Source: CAD feature listing. Evaluate the final solid. Frame: model axes, mm. A direction names the side the tool comes from. Round coordinates to 2 decimals unless told otherwise and drop trailing zeros. Order: outer loops, then holes, each group sorted by start corner. A loop starts at its lowest first (then second) coordinate and runs counter-clockwise, first axis right, second up. Notation, with made-up numbers: (-6.5, -3) - (15.5, -3) arc R12 ccw to (15.5, 2) - close; hole circle Ø8 at (60, -32). An arc over 180 degrees is marked (long way). Use one line per item in the form item = value. Start each with the question number.
Q1. Cut plane A-A, the plane x = 48.2. Return the cut outline in (y, z), and give its area (3 significant figures).
Q2. Ray query, line 1 (Z direction, x = -5.3, y = 27.5); line 2 (X direction, y = 44.25, z = -9.6) (3 decimals); line 3 (Y direction, x = 5.5, z = -8). Return the intervals inside material, ascending. Write a range as [from, to].
Q3. Cut plane B-B, the plane x = 28. Return the cut outline in (y, z), and give its area (3 significant figures).
Q4. Draft query along X for faces 1 (the cylindrical face through (45.8, 26.82, -4.71)), 2 (the cylindrical face through (-2.9, 26.82, -14.31)), 3 (the flat face through (-8, 27, -3)), 4 (the flat face through (22, 38.7, -10)). Return one class per face: released by +X, released by -X, zero draft, split by the parting line, or undercut.
Q5. Cut plane D-D, the plane y = 23. Return the cut outline in (x, z), and give its area (3 significant figures).
Q6. Pin query (flat end, axial travel): pin 1 Ø1.7 at (x, z) = (10.725, -9.6) entering from +Y; pin 2 Ø2.5 at (y, z) = (37, -13) entering from +X; pin 3 Ø2 at (y, z) = (22.5, -4.5) entering from -X. Return the tip coordinate at first contact, or that it passes through.
Q7. Set-up query: faces 5 (the flat face through (16, 40.2, -13)), 6 (the flat face through (35.175, 37.5, -3.7)), 7 (the flat face through (47, 28.3, -10)). Return all of +Z, -Z, +X, -X, +Y, -Y with unobstructed straight access to the full face (end or side cutting, diameter ignored); none if empty.
from build123d import *

# Parameters (mm, degrees)
SKETCH_1_W             = 42.9
SKETCH_1_H             = 19.2
EXTRUDE_1_DEPTH        = 35.7
EXTRUDE_3_DEPTH        = 3
SKETCH_5_R             = 7.2
EXTRUDE_4_DEPTH        = 1.5
SKETCH_6_R             = 5.76
EXTRUDE_5_DEPTH        = 0.3
CUT_EXTRUDE_START      = -0.3
CUT_EXTRUDE_3_DEPTH    = 0.3
EXTRUDE_6_DEPTH        = 8
FILLET_1_R             = 2
FILLET_2_R             = 2
CUT_EXTRUDE_4_DEPTH    = 62.321611199
FILLET_1_OF_MIRROR_2_R = 2
FILLET_2_OF_MIRROR_2_R = 2
SKETCH_10_R            = 2.88
EXTRUDE_7_DEPTH        = 6
SKETCH_11_R            = 1.44
CUT_EXTRUDE_5_DEPTH    = 6


with BuildPart() as part:
    # Sketch 1 → Extrude 1 (new body)
    with BuildSketch(Plane(origin=(0, 0, 0), x_dir=(1, 0, 0), z_dir=(0, 1, 0))):
        with Locations((21.45, 9.6)):
            Rectangle(SKETCH_1_W, SKETCH_1_H)
    extrude(amount=EXTRUDE_1_DEPTH)

    # Sketch 2 → Extrude 3 (add)
    with BuildSketch(Plane(origin=(0, 35.7, 0), x_dir=(1, 0, 0), z_dir=(0, 1, 0))):
        with BuildLine():
            Line((35.175, 1), (35.175, 3.875))
            ThreePointArc((35.175, 3.875), (40.9, 9.6), (35.175, 15.325))
            Line((35.175, 15.325), (35.175, 18.2))
            Line((35.175, 18.2), (14.991145802, 18.2))
            ThreePointArc((14.991145802, 18.2), (1.125, 9.6), (14.991145802, 1))
            Line((14.991145802, 1), (35.175, 1))
        make_face()
    extrude(amount=EXTRUDE_3_DEPTH)

    # Sketch 5 → Extrude 4 (add)
    with BuildSketch(Plane(origin=(0, 38.7, 0), x_dir=(1, 0, 0), z_dir=(0, 1, 0))):
        with Locations(Location((10.725, 9.6, 0), (0, 0, 270))):
            Circle(SKETCH_5_R)
    extrude(amount=EXTRUDE_4_DEPTH)

    # Sketch 6 → Extrude 5 (add)
    with BuildSketch(Plane(origin=(0, 40.2, 0), x_dir=(1, 0, 0), z_dir=(0, 1, 0))):
        with Locations(Location((10.725, 9.6, 0), (0, 0, 270))):
            Circle(SKETCH_6_R)
    extrude(amount=EXTRUDE_5_DEPTH)

    # Sketch 4 → Cut-Extrude 3 (cut)
    with BuildSketch(Plane(origin=(0, 38.7, 0), x_dir=(1, 0, 0), z_dir=(0, 1, 0)).offset(CUT_EXTRUDE_START)):
        with BuildLine():
            Line((35.175, 15.325), (35.175, 3.875))
            ThreePointArc((35.175, 3.875), (40.9, 9.6), (35.175, 15.325))
        make_face()
    extrude(amount=CUT_EXTRUDE_3_DEPTH, mode=Mode.SUBTRACT)

    # Sketch 8 → Extrude 6 (add)
    with BuildSketch(Plane(origin=(42.9, 0, 0), x_dir=(0, 0, -1), z_dir=(1, 0, 0))):
        Polygon((19.2, 26.8), (19.2, 28.3), (0, 28.3), (0, 25.3), (19.2, 25.3), align=None)
    extrude_6 = extrude(amount=EXTRUDE_6_DEPTH)

    # Fillet 1
    fillet_1_edges = [part.edges().sort_by_distance(p)[0] for p in [
        (50.9, 26.8, 0),
    ]]
    fillet(fillet_1_edges, radius=FILLET_1_R)

    # Fillet 2
    fillet_2_edges = [part.edges().sort_by_distance(p)[0] for p in [
        (50.9, 26.8, -19.2),
    ]]
    fillet(fillet_2_edges, radius=FILLET_2_R)

    # Sketch 9 → Cut-Extrude 4 (cut, through all)
    with BuildSketch(Plane(origin=(0, 28.3, 0), x_dir=(1, 0, 0), z_dir=(0, 1, 0))):
        with BuildLine():
            Line((50.381742423, 5.8), (50.9, 5.8))
            Line((50.9, 5.8), (50.9, 3.8))
            Line((50.9, 3.8), (50.381742423, 3.8))
            ThreePointArc((50.381742423, 3.8), (45.8, 4.8), (50.381742423, 5.8))
        make_face()
        with BuildLine():
            Line((50.381742423, 15.4), (50.9, 15.4))
            Line((50.9, 15.4), (50.9, 13.4))
            Line((50.9, 13.4), (50.381742423, 13.4))
            ThreePointArc((50.381742423, 13.4), (45.8, 14.4), (50.381742423, 15.4))
        make_face()
    cut_extrude_4 = extrude(amount=-CUT_EXTRUDE_4_DEPTH, mode=Mode.SUBTRACT)

    # Mirror 2: Extrude 6, Cut-Extrude 4 across plane
    add(extrude_6.mirror(Plane(origin=(21.45, 0, 0), x_dir=(0, 0, 1), z_dir=(1, 0, 0))))
    add(cut_extrude_4.mirror(Plane(origin=(21.45, 0, 0), x_dir=(0, 0, 1), z_dir=(1, 0, 0))), mode=Mode.SUBTRACT)

    # Fillet 1 of Mirror 2
    fillet_1_of_mirror_2_edges = [part.edges().sort_by_distance(p)[0] for p in [
        (-8, 26.8, 0),
    ]]
    fillet(fillet_1_of_mirror_2_edges, radius=FILLET_1_OF_MIRROR_2_R)

    # Fillet 2 of Mirror 2
    fillet_2_of_mirror_2_edges = [part.edges().sort_by_distance(p)[0] for p in [
        (-8, 26.8, -19.2),
    ]]
    fillet(fillet_2_of_mirror_2_edges, radius=FILLET_2_OF_MIRROR_2_R)

    # Sketch 10 → Extrude 7 (add)
    with BuildSketch(Plane(origin=(0, 40.5, 0), x_dir=(1, 0, 0), z_dir=(0, 1, 0))):
        with Locations(Location((10.725, 9.6, 0), (0, 0, 270))):
            Circle(SKETCH_10_R)
    extrude(amount=EXTRUDE_7_DEPTH)

    # Sketch 11 → Cut-Extrude 5 (cut)
    with BuildSketch(Plane(origin=(0, 46.5, 0), x_dir=(1, 0, 0), z_dir=(0, 1, 0))):
        with Locations(Location((10.725, 9.6, 0), (0, 0, 270))):
            Circle(SKETCH_11_R)
    extrude(amount=-CUT_EXTRUDE_5_DEPTH, mode=Mode.SUBTRACT)


solid = part.part
Completed:
q1.outline = (25.3, -19.2) - (28.3, -19.2) - (28.3, -16.8) - (25.3, -16.8) - close; (25.3, -12) - (28.3, -12) - (28.3, -7.2) - (25.3, -7.2) - close; (25.3, -2.4) - (28.3, -2.4) - (28.3, 0) - (25.3, 0) - close
q1.area = 28.8 mm2
q2.line_1 = [-19.2, -16.8], [-12, -7.2], [-2.4, 0]
q2.line_2 = [7.845, 9.285], [12.165, 13.605]
q2.line_3 = [0, 40.5]
q3.outline = (0, -19.2) - (35.7, -19.2) - (35.7, -18.2) - (38.7, -18.2) - (38.7, -1) - (35.7, -1) - (35.7, 0) - (0, 0) - close
q3.area = 737 mm2
q4.face_1 = undercut
q4.face_2 = undercut
q4.face_3 = released by -X
q4.face_4 = zero draft
q5.outline = (0, -19.2) - (42.9, -19.2) - (42.9, 0) - (0, 0) - close
q5.area = 824 mm2
q6.pin_1 = 40.5
q6.pin_2 = 40.48
q6.pin_3 = 0
q7.face_5 = +Y
q7.face_6 = +X, +Y
q7.face_7 = +Z, -Z, +X, +Y
